Answer from the drawing. Dimensions are ordinates in mm from the lowest x, y and z of the part. Coordinates: 2 decimals unless noted, no trailing zeros. Write each loop counter-clockwise with the first axis right and the second up, starting at its lowest first coordinate (ties: lowest second). Pieces come first, ordered by that corner, then holes.
(1) Section C-C on x = 12 is taken. Write down the section's boundary in (y, z), then the cut area to 3 significant figures.
(2) Section B-B on x = 15 is taken. Write down the section's boundary in (y, z).
(3) Given pin 1 (7 mm diameter, centred on x = 12, z = 8.5, fed in from -Y); pin 2 (3 mm diameter, centred on x = 7.5, y = 3, fed in from -Z) (1 decimal), each flat-ended and moving along its own axis, determine where each tip first touches the part or whether it passes through.
(4) Section D-D on y = 1.5 is taken. Write down the section's boundary in (x, z), then the cut area to 3 significant figures.
(5) The mould has two halves that part along X. Classify the marked faces 1, 2, 3 and 4: +X half, -X half, draft (parallel to the pull), parting line (faces both ways), or undercut.
(6) Find the intervals of material crossed by probe 1 along X at (y, z) = (3.4, 5); probe 2 along Y at (x, z) = (22.75, 12.5); probe 3 along Z at (x, y) = (14.25, 3.7), in increasing order.
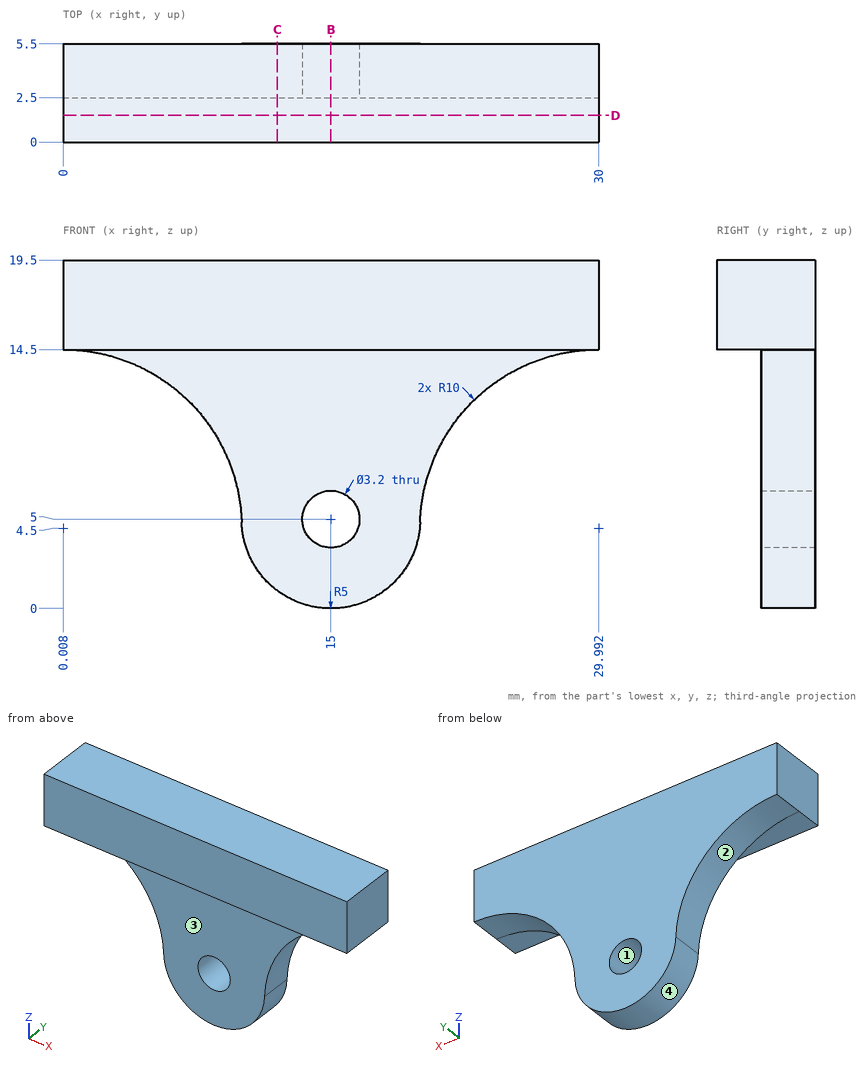
Response:
1. outline: (0, 14.5) - (2.5, 14.5) - (2.5, 1) - (5.5, 1) - (5.5, 19.5) - (0, 19.5) - close
1. area: 68.0 mm2
2. outline: (0, 14.5) - (2.5, 14.5) - (2.5, 6.6) - (5.5, 6.6) - (5.5, 19.5) - (0, 19.5) - close; (2.5, 0) - (5.5, 0) - (5.5, 3.4) - (2.5, 3.4) - close
3. pin 1: stops at y = 2.5
3. pin 2: stops at z = 8.9
4. outline: (0, 14.5) - (30, 14.5) - (30, 19.5) - (0, 19.5) - close
4. area: 150 mm2
5. face 1: undercut
5. face 2: -X half
5. face 3: draft
5. face 4: parting line
6. probe 1: x = 10 to 13.4, 16.6 to 20
6. probe 2: y = 2.5 to 5.5
6. probe 3: z = 0.06 to 3.59, 6.41 to 19.5
